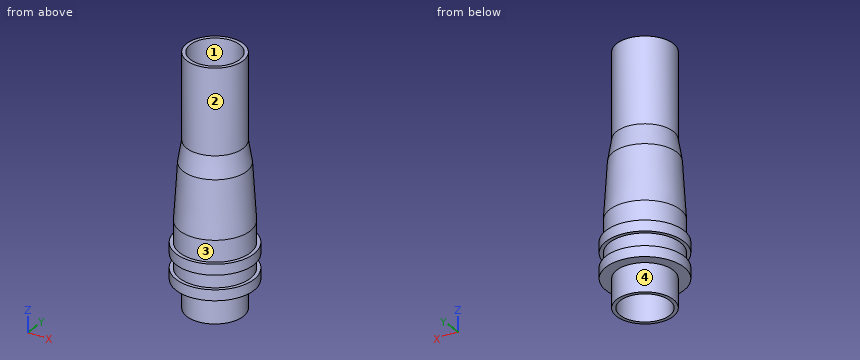
```python
from build123d import *

# Parameters (mm, degrees)
F3_D = 7


with BuildPart() as f1:
    # F0 (on Front) → F1 (revolve)
    with BuildSketch(Plane.XZ):
        Polygon((-4, 0), (0, 0), (0, 35), (-4, 35), (-4, 23), (-4.5, 20), (-5, 12), (-5, 9), (-5.5, 9), (-5.5, 7.5), (-5, 7.5), (-5, 5.5), (-5.5, 5.5), (-5.5, 4), (-4, 4), align=None)
    revolve(axis=Axis((0, 0, 17.5), (0, 0, 1)))

    # F3 (through all)
    with Locations(Plane(origin=(0, 0, 0), x_dir=(1, 0, 0), z_dir=(0, 0, -1))):
        with Locations((0, 0)):
            Hole(F3_D / 2)


solid = f1.part
```
CAD build for the part. Positions are in the model's coordinates, mm. Face numbers are marked on the shaded views. A direction names the side the tool comes from. Round coordinates to 2 decimals unless told otherwise and drop trailing zeros. Write each loop counter-clockwise with the first axis right and the second up, starting at its lowest first coordinate (ties: lowest second). Pieces come first, ordered by that corner, then holes. Notation, with made-up numbers: (15, 33.25) - (48, 33.25) arc R19 ccw to (48, 62.25) - close; hole circle Ø7 at (-33.75, -22.75). An arc over 180 degrees is marked (long way). Write item = value, one per line. Start each with the question number.
Q1. Band-saw the part on C-C (z = 32.5). Give the cut face in (x, y), then the cut area to 3 significant figures.
Q2. Probe L1, parallel to Y at x = 0, z = 8; L2, parallel to Y at x = 0, z = 27.5; L3, parallel to X at y = 1.75, z = 28.5. List the from-to ranges inside material, lowest first. Write a range as from..to.
Q3. Band-saw the part on D-D (z = 17.5). Give the cut face in (x, y).
Q4. Which spindle directions (+Z, -Z, +X, -X, +Y, -Y) get a long thin tool onto all of the face, cutting with end or side? Do the marked faces 3 and 4. Say none if no direction does.
Q5. Drop flat-ended pins along their axis: pin 1 (6 mm diameter, centred on x = -1, z = 23, fed in from -Y); pin 2 (4 mm diameter, centred on y = -1.5, z = 14, fed in from -X); pin 3 (2 mm diameter, centred on y = 1, z = 20.5, fed in from +X). Give the stop position or say it passes through.
Q6. Mould opens along Y. For the marked faces 1 and 2 say: pulls with the +Y half, pulls with the -Y half, needs draft (parallel to the pull), parting line crosses it, or undercut.
Answers below:
q1.outline = circle Ø8 at (0, 0); hole circle Ø7 at (0, 0)
q1.area = 11.8 mm2
q2.L1 = -5.5..-3.5, 3.5..5.5
q2.L2 = -4..-3.5, 3.5..4
q2.L3 = -3.6..-3.03, 3.03..3.6
q3.outline = circle Ø9.31 at (0, 0); hole circle Ø7 at (0, 0)
q4.face_3 = +Z
q4.face_4 = -Z
q5.pin_1 = -4.48
q5.pin_2 = -4.97
q5.pin_3 = 4.5
q6.face_1 = undercut
q6.face_2 = parting line crosses it
